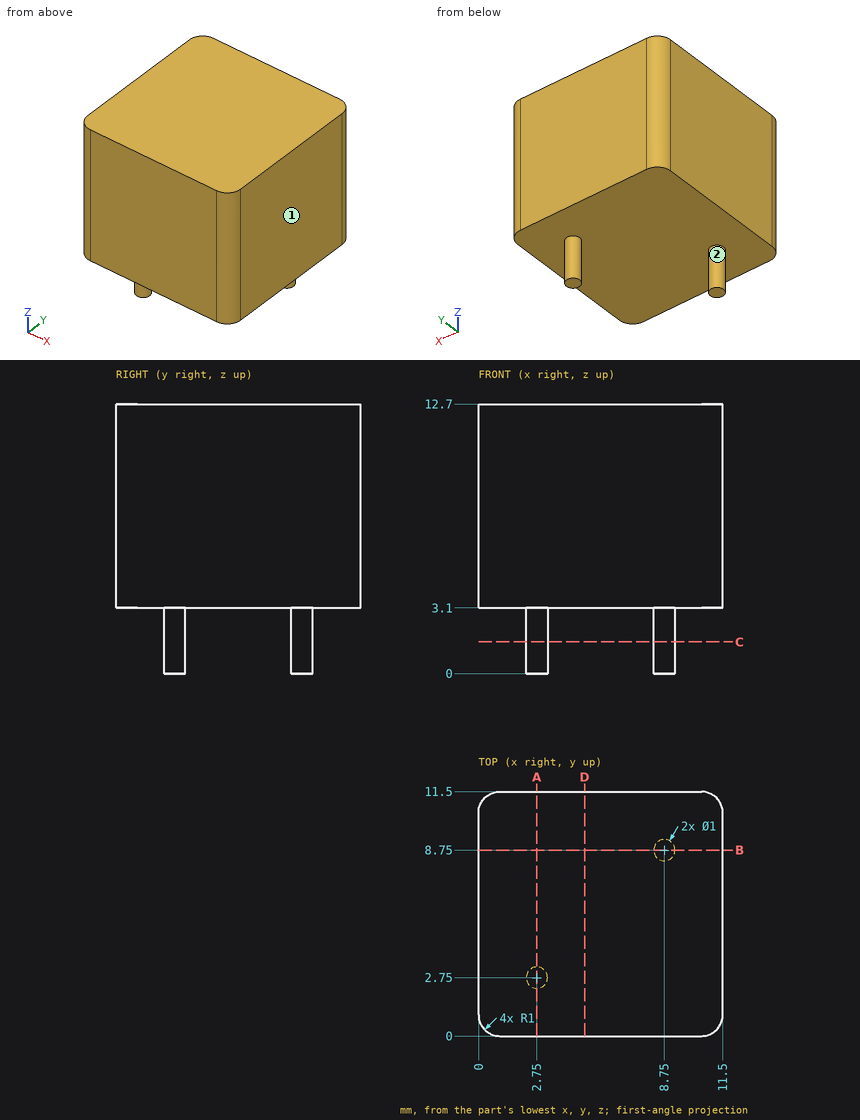
Check sheet for the drawn part. Datum: minimum x, y, z corner. Units: mm. A direction names the side the tool comes from. Round coordinates to 2 decimals unless told otherwise and drop trailing zeros. Order: outer loops, then holes, each group sorted by start corner. A loop starts at its lowest first (then second) coordinate and runs counter-clockwise, first axis right, second up. Notation, with made-up numbers: M -34,18 L 9,18 A12 cw 9,35 Z; hole C 67.5,38 d2. An arc over 180 degrees is marked long. Write each question's results on one line, items separated by ' | '. Start each with the question number.
1. Cross-section at D-D on x = 5. Record the boundary of the cut face in (y, z), plus the area to 3 significant figures.
2. Cross-section at A-A on x = 2.75. Record the boundary of the cut face in (y, z), plus the area to 4 significant figures.
3. Material ranges on L1, parallel to Z at x = 8.25, y = 9; L2, parallel to Y at x = 0.75, z = 9.75, recorded low to high. Write a range as from..to.
4. Go/stop test with flat-tipped pins: P1, Ø4, axis at x = 4, y = 7.5, coming from the -Z side; P2, Ø2, axis at x = 3.5, z = 2.5, coming from the +Y side. Record where each tip stops, or that it passes through.
5. Cross-section at B-B on y = 8.75. Record the boundary of the cut face in (x, z).
6. Cross-section at C-C on z = 1.5. Record the boundary of the cut face in (x, y), plus the area to 3 significant figures.
7. Set-up check for the marked faces 1 and 2: record each of +Z, -Z, +X, -X, +Y, -Y from which the full face is reachable in a straight line by a thin tool's end or side.
Resolved:
1) outline: M 0,3.1 L 11.5,3.1 L 11.5,12.7 L 0,12.7 Z | area: 110 mm2
2) outline: M 0,3.1 L 2.25,3.1 L 2.25,0 L 3.25,0 L 3.25,3.1 L 11.5,3.1 L 11.5,12.7 L 0,12.7 Z | area: 113.5 mm2
3) L1: 3.1..12.7 | L2: 0.03..11.47
4) P1: z = 3.1 | P2: y = 11.5
5) outline: M 0,3.1 L 8.25,3.1 L 8.25,0 L 9.25,0 L 9.25,3.1 L 11.5,3.1 L 11.5,12.7 L 0,12.7 Z
6) outline: C 2.75,2.75 d1; C 8.75,8.75 d1 | area: 1.57 mm2
7) face 1: +Z, -Z, +X, +Y, -Y | face 2: -Z
